Geometry check sheet. Reference: drawing and pictorial views, mm from the part's lowest x, y, z. A direction names the side the tool comes from. Coordinates: 2 decimals unless noted, no trailing zeros. Write each loop counter-clockwise with the first axis right and the second up, starting at its lowest first coordinate (ties: lowest second). Pieces come first, ordered by that corner, then holes. Notation, with made-up numbers: (-23.75, 55) -> (-4.75, 55) arc R23 cw to (-4.75, 72) -> close; hole circle Ø5 at (-13, 39.25). An arc over 180 degrees is marked (long way). Put each result on its own line as item: value.
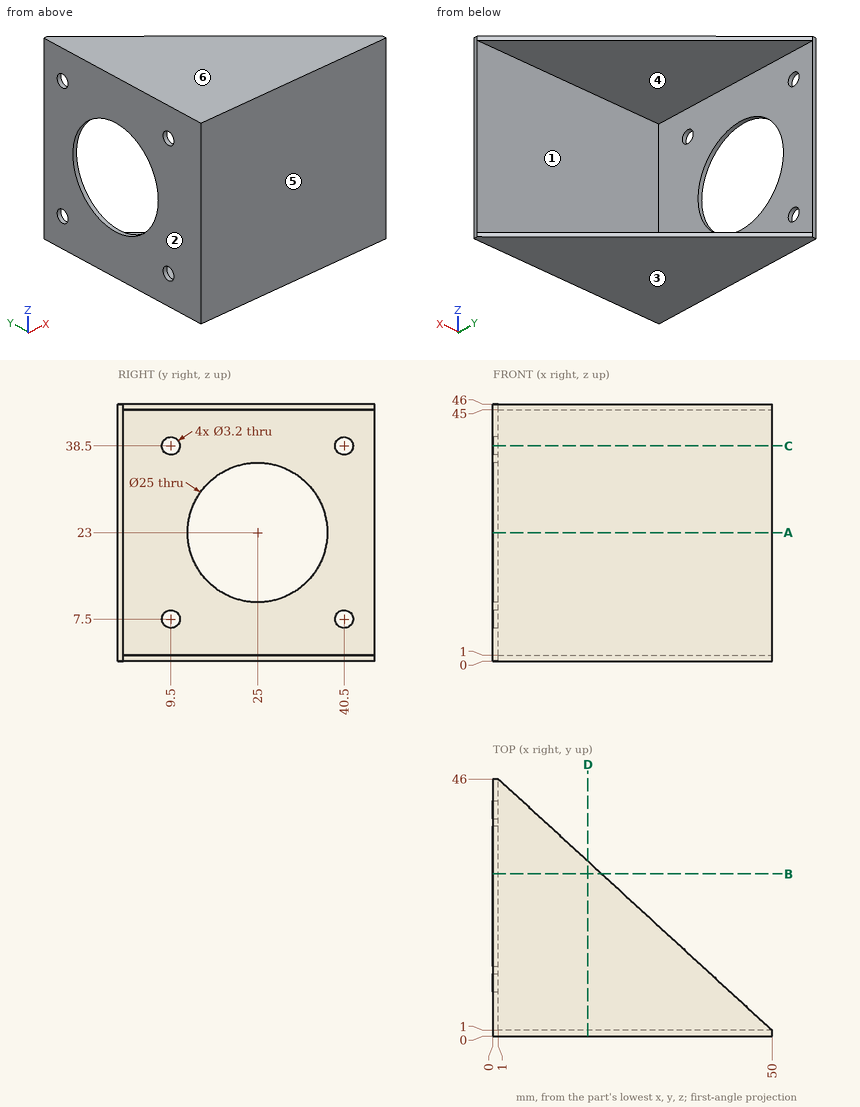
Q1. Cross-section at B-B (y = 29). Record the cut outline in (x, z), plus the area to 3 significant figures.
Recorded:
outline: (0, 0) -> (19.51, 0) -> (19.51, 1) -> (1, 1) -> (1, 11.16) -> (0, 11.16) -> close; (0, 34.84) -> (1, 34.84) -> (1, 45) -> (19.51, 45) -> (19.51, 46) -> (0, 46) -> close
area: 59.3 mm2
Q2. Tool access check on the marked faces 1 and 2. Record the directions out of +Z, -Z, +X, -X, +Y, -Y that give a thin tool (end or side, any length) a straight path to the whole face; none if there is none.
Recorded:
face 1: +X, +Y
face 2: +Z, -Z, -X, +Y, -Y
Q3. Material ranges on line 1 along Y through (x, z) = (0.4, 38.5); line 2 along Z through (x, y) = (8, 22); line 3 along Z through (x, y) = (0.45, 25), recorded low to high.
Recorded:
line 1: y = 0 to 7.9, 11.1 to 38.9, 42.1 to 46
line 2: z = 0 to 1, 45 to 46
line 3: z = 0 to 10.5, 35.5 to 46
Q4. Cross-section at D-D (x = 17). Record the cut outline in (y, z).
Recorded:
outline: (0, 0) -> (31.31, 0) -> (31.31, 1) -> (1, 1) -> (1, 45) -> (31.31, 45) -> (31.31, 46) -> (0, 46) -> close
Q5. Depth check by flat-ended pin: P1, Ø1, axis at x = 25.5, z = 5.5, coming from the +Y side; P2, Ø2, axis at y = 38, z = 8.5, coming from the +X side. Enter the tip coordinate at first touch or a pass-through.
Recorded:
P1: stops at y = 1
P2: stops at x = 1
Q6. Cross-section at C-C (z = 38.5). Record the cut outline in (x, y), plus the area to 3 significant figures.
Recorded:
outline: (0, 0) -> (50, 0) -> (50, 1) -> (1, 1) -> (1, 7.9) -> (0, 7.9) -> close; (0, 11.1) -> (1, 11.1) -> (1, 38.9) -> (0, 38.9) -> close; (0, 42.1) -> (1, 42.1) -> (1, 46) -> (0, 46) -> close
area: 88.6 mm2
Q7. Mould release check, pull along Z, two halves, no side actions. Record for the marked faces 3, 4, 5 and 6: released by +Z, released by -Z, zero draft, split by the parting line, or undercut.
Recorded:
face 3: released by -Z
face 4: undercut
face 5: zero draft
face 6: released by +Z
Q8. Cross-section at A-A (z = 23). Record the cut outline in (x, y).
Recorded:
outline: (0, 0) -> (50, 0) -> (50, 1) -> (1, 1) -> (1, 12.5) -> (0, 12.5) -> close; (0, 37.5) -> (1, 37.5) -> (1, 46) -> (0, 46) -> close
